CAD build for the part. Positions are in the model's coordinates, mm. Face numbers are marked on the shaded views. A direction names the side the tool comes from. Give positions to 0.01 mm unless a question says otherwise; leave off trailing zeros. Loops run counter-clockwise (first coordinate to the right, second up) from the corner with the lowest first, then second, coordinate; pieces in that order, holes last. Notation, with made-up numbers: (11, 44.5) - (60, 44.5) arc R11 ccw to (60, 50.5) - close; hole circle Ø4 at (34, 9). An arc over 180 degrees is marked (long way). Return JSON: item names as keys, results as strings.
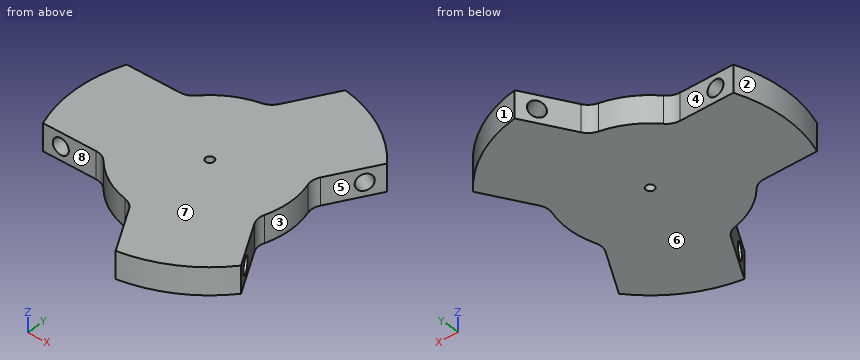
from build123d import *

# Parameters (mm, degrees)
SKIZZE1_R                       = 25
AUFSATZ_LINEAR_AUSTRAGEN1_DEPTH = 5
SCHNITT_LINEAR_AUSTRAGEN1_DEPTH = 36.707142143
SKIZZE3_R                       = 1.5
SCHNITT_LINEAR_AUSTRAGEN2_DEPTH = 43.256635771
KREISMUSTER1_COUNT              = 3
SKIZZE6_R                       = 0.78
SCHNITT_LINEAR_AUSTRAGEN5_DEPTH = 36.497057468
VERRUNDUNG1_R                   = 3


with BuildPart() as part:
    # Skizze1 → Aufsatz-Linear austragen1 (new body)
    with BuildSketch(Plane.XY):
        Circle(SKIZZE1_R)
    extrude(amount=AUFSATZ_LINEAR_AUSTRAGEN1_DEPTH)

    # Skizze2 → Schnitt-Linear austragen1 (cut, through all)
    with BuildSketch(Plane.XY.offset(5)):
        with BuildLine():
            Line((19.456132424, 15.699009877), (13.794228634, 5.892304845))
            ThreePointArc((13.794228634, 5.892304845), (15, 0), (13.794228634, -5.892304845))
            Line((13.794228634, -5.892304845), (19.456132424, -15.699009877))
            ThreePointArc((19.456132424, -15.699009877), (25, 0), (19.456132424, 15.699009877))
        make_face()
        with BuildLine():
            Line((-23.323807579, 9), (-12, 9))
            ThreePointArc((-12, 9), (-7.5, 12.990381057), (-1.794228634, 14.892304845))
            Line((-1.794228634, 14.892304845), (3.867675156, 24.699009877))
            ThreePointArc((3.867675156, 24.699009877), (-12.5, 21.650635095), (-23.323807579, 9))
        make_face()
        with BuildLine():
            Line((3.867675156, -24.699009877), (-1.794228634, -14.892304845))
            ThreePointArc((-1.794228634, -14.892304845), (-7.5, -12.990381057), (-12, -9))
            Line((-12, -9), (-23.323807579, -9))
            ThreePointArc((-23.323807579, -9), (-12.5, -21.650635095), (3.867675156, -24.699009877))
        make_face()
    extrude(amount=-SCHNITT_LINEAR_AUSTRAGEN1_DEPTH, mode=Mode.SUBTRACT)

    # Skizze3 → Schnitt-Linear austragen2 (cut, through all)
    with BuildSketch(Plane(origin=(0, 9, 0), x_dir=(1, 0, 0), z_dir=(0, 1, 0))):
        with Locations(Location((-20, -2.5, 0), (0, 0, 270))):
            Circle(SKIZZE3_R)
    schnitt_linear_austragen2 = extrude(amount=-SCHNITT_LINEAR_AUSTRAGEN2_DEPTH, mode=Mode.SUBTRACT)

    # Kreismuster1: Schnitt-Linear austragen2 ×3 about axis
    kreismuster1_axis = Axis((0, 0, 5), (0, 0, -1))
    for i in range(1, KREISMUSTER1_COUNT):
        add(schnitt_linear_austragen2.rotate(kreismuster1_axis, i * 360 / KREISMUSTER1_COUNT), mode=Mode.SUBTRACT)

    # Skizze6 → Schnitt-Linear austragen5 (cut, through all)
    with BuildSketch(Plane.XY.offset(5)):
        Circle(SKIZZE6_R)
    extrude(amount=-SCHNITT_LINEAR_AUSTRAGEN5_DEPTH, mode=Mode.SUBTRACT)

    # Verrundung1
    verrundung1_edges = [part.edges().sort_by_distance(p)[0] for p in [
        (-1.794228634, 14.892304845, 2.5),
        (-12, 9, 2.5),
        (-12, -9, 2.5),
        (-1.794228634, -14.892304845, 2.5),
        (13.794228634, -5.892304845, 2.5),
        (13.794228634, 5.892304845, 2.5),
    ]]
    fillet(verrundung1_edges, radius=VERRUNDUNG1_R)


solid = part.part
1. Drop a flat-ended pin along its axis: P1, Ø1.5, axis at x = -16.5, z = 4.5, coming from the -Y side. Give the stop position or say it passes through.
Values follow:
{"P1": "stops at y = -9"}
2. Cut at D-D, the plane x = 0. Write the cut outline in (y, z), plus the area to 3 significant figures.
Values follow:
{"outline": "(-18, 0) - (-0.78, 0) - (-0.78, 5) - (-18, 5) - close; (0.78, 0) - (18, 0) - (18, 5) - (0.78, 5) - close", "area": "172 mm²"}
3. Drill centre lines: probe 1 along Y at (x, z) = (-20.5, 0.85); probe 2 along Y at (x, z) = (0, 2.2); probe 3 along Y at (x, z) = (7.5, 1.45). Where is each one in solid material? Low to high.
Values follow:
{"probe 1": "y = -9 to 9", "probe 2": "y = -18 to -0.78, 0.78 to 18", "probe 3": "y = -23.85 to -20, -17.53 to 17.53, 20 to 23.85"}
4. Cut at A-A, the plane y = 0. Write the cut outline in (x, z), plus the area to 3 significant figures.
Values follow:
{"outline": "(-25, 0) - (-0.78, 0) - (-0.78, 5) - (-25, 5) - close; (0.78, 0) - (15, 0) - (15, 5) - (0.78, 5) - close; hole circle Ø3 at (-20, 2.5)", "area": "185 mm²"}
5. Cut at C-C, the plane x = -20. Write the cut outline in (y, z).
Values follow:
{"outline": "(-9, 0) - (9, 0) - (9, 1) - (-9, 1) - close; (-9, 4) - (9, 4) - (9, 5) - (-9, 5) - close"}
6. Pull direction Y, two halves, no side cores. Call the marked faces 1, 2 and 3: +Y half, -Y half, draft (parallel to the pull), parting line (faces both ways), or undercut.
Values follow:
{"face 1": "+Y half", "face 2": "parting line", "face 3": "undercut"}
7. Which spindle directions (+Z, -Z, +X, -X, +Y, -Y) get a long thin tool onto all of the face, cutting with end or side? Do the marked faces 4, 5, 6, 7 and 8. Say none if no direction does.
Values follow:
{"face 4": "+Z, -Z, -X, +Y", "face 5": "+Z, -Z, +X", "face 6": "-Z, +X, -X, +Y, -Y", "face 7": "+Z, +X, -X, +Y, -Y", "face 8": "+Z, -Z, -X, -Y"}
8. Cut at B-B, the plane z = 1.8. Give the number of separate pieces and of enclosed holes in the cut face, plus the area to 3 significant figures.
Values follow:
{"separate pieces": "4", "enclosed holes": "1", "area": "1,130 mm²"}
